For this review, use the dimensioned drawing (mm, ordinates from the lowest corner) and the shaded views. Give positions to 0.01 mm unless a question says otherwise; leave off trailing zeros. Write each loop counter-clockwise with the first axis right and the second up, starting at its lowest first coordinate (ties: lowest second). Pieces come first, ordered by that corner, then holes. Notation, with made-up numbers: M 27.5,-25.75 L 76.5,-25.75 A14 ccw 76.5,-5.75 Z; hole C 56.25,21.5 d10. An arc over 180 degrees is marked long. One line per item, written item: value. Start each with the question number.
Item 1: Consider section C-C, the plane z = 225.5. Write out the cut boundary in (x, y).
Item 2: Consider section A-A, the plane z = 17. Write out the cut boundary in (x, y) (1 decimal).
Item 3: Clearance check with flat-ended pins moving along their axes: pin 1 Ø4 at (y, z) = (3, 169.5) entering from +X; pin 2 Ø3 at (y, z) = (7.5, 179.5) entering from -X; pin 3 Ø2 at (x, y) = (44, 4) entering from +Z; pin 4 Ø12 at (x, z) = (54, 137.5) entering from +Y. State where each tip first meets the part, or that it passes through.
Item 4: Consider section D-D, the plane x = 10. Write out the cut boundary in (y, z) (1 decimal), and give its area (3 significant figures).
Item 5: To check wall thickness, follow probe 1 along X at (y, z) = (4.25, 36) (1 decimal); probe 2 along X at (y, z) = (9.5, 126.5); probe 3 along X at (y, z) = (2.75, 58.5). State the ranges of each line that lie inside material, in increasing order.
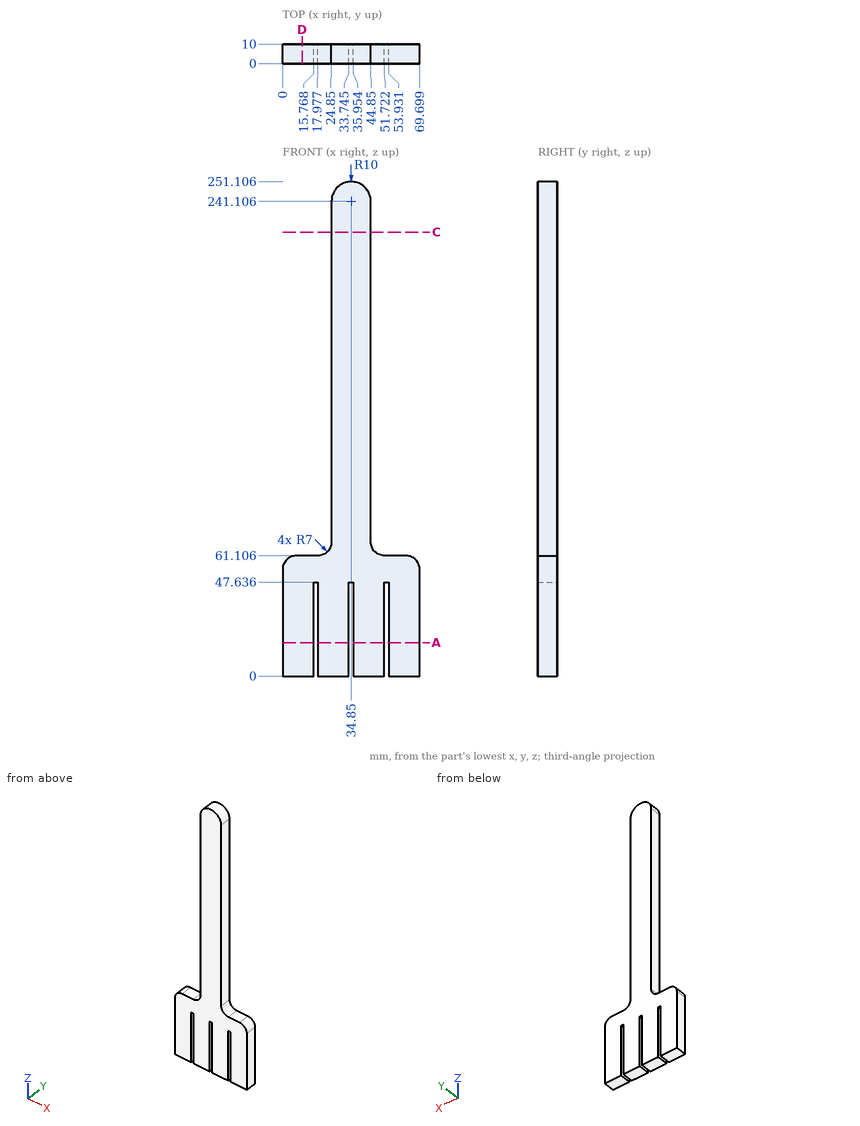
Model answer:
1. outline: M 24.85,0 L 44.85,0 L 44.85,10 L 24.85,10 Z
2. outline: M 0,0 L 15.8,0 L 15.8,10 L 0,10 Z; M 18,0 L 33.7,0 L 33.7,10 L 18,10 Z; M 36,0 L 51.7,0 L 51.7,10 L 36,10 Z; M 53.9,0 L 69.7,0 L 69.7,10 L 53.9,10 Z
3. pin 1: stops at x = 44.85
3. pin 2: stops at x = 24.85
3. pin 3: stops at z = 246.9
3. pin 4: passes through
4. outline: M 0,0 L 10,0 L 10,61.1 L 0,61.1 Z
4. area: 611 mm2
5. probe 1: x = 0 to 15.8, 18 to 33.7, 36 to 51.7, 53.9 to 69.7
5. probe 2: x = 24.85 to 44.85
5. probe 3: x = 1.55 to 68.15
